Could you check a few things on this drawing? It's one solid part, dimensions in mm from its lowest x, y, z. A direction names the side the tool comes from. Give positions to 0.01 mm unless a question says otherwise; leave off trailing zeros. Loops run counter-clockwise (first coordinate to the right, second up) from the corner with the lowest first, then second, coordinate; pieces in that order, holes last. Notation, with made-up numbers: M 74.25,68 L 124.25,68 A20 ccw 124.25,82 Z; hole C 85.25,44.25 d4. An arc over 180 degrees is marked long. Answer as a JSON object with one key per item and string values.
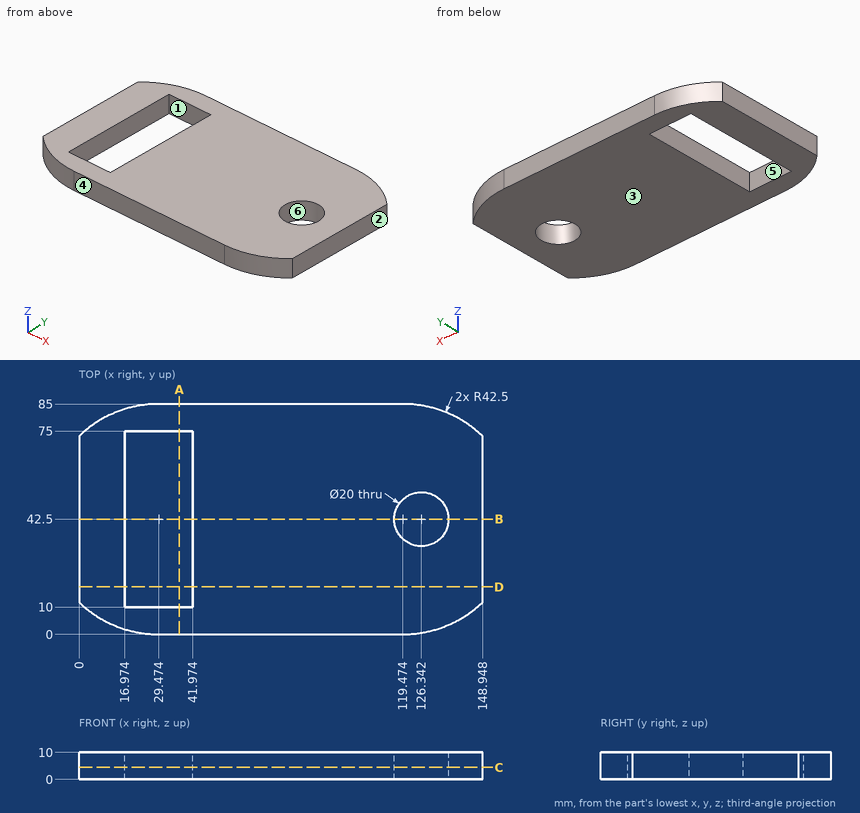
1) Will this pin go through, and if not, where does the flat tip stop? pin 1 Ø3 at (y, z) = (41.5, 7.5) entering from -X.
Answer list:
{"pin 1": "x = 0"}
2) Suppose I cut it at A-A, the plane x = 37. Write out the boundary of the cut face in (y, z).
Answer list:
{"outline": "M 0,0 L 10,0 L 10,10 L 0,10 Z; M 75,0 L 85,0 L 85,10 L 75,10 Z"}
3) Please list where these lines run through material, in increasing order: line 1 along X through (y, z) = (73, 1.75); line 2 along Y through (x, z) = (23, 3.25); line 3 along X through (y, z) = (48.5, 3) (1 decimal). Write a range as from..to.
Answer list:
{"line 1": "0..16.97, 41.97..148.95", "line 2": "0.5..10, 75..84.5", "line 3": "0..17, 42..118.3, 134.3..148.9"}
4) Suppose I cut it at D-D, the plane y = 17.5. Write out the boundary of the cut face in (x, z).
Answer list:
{"outline": "M 0,0 L 16.97,0 L 16.97,10 L 0,10 Z; M 41.97,0 L 148.95,0 L 148.95,10 L 41.97,10 Z"}
5) Suppose I cut it at C-C, the plane z = 4.5. Write out the boundary of the cut face in (x, y).
Answer list:
{"outline": "M 0,11.88 A42.5 ccw 29.47,0 L 119.47,0 A42.5 ccw 148.95,11.88 L 148.95,73.12 A42.5 ccw 119.47,85 L 29.47,85 A42.5 ccw 0,73.12 Z; hole M 16.97,10 L 41.97,10 L 41.97,75 L 16.97,75 Z; hole C 126.34,42.5 d20"}
6) For the marked faces 1 and 2, which set-ups out of +Z, -Z, +X, -X, +Y, -Y let a thin tool reach every point of the face, with its end or its side?
Answer list:
{"face 1": "+Z, -Z", "face 2": "+Z, -Z, +X, +Y, -Y"}
7) If we mould it in two halves opening along Y, with no side actions, what happens to the marked faces 3, 4, 5 and 6? For each: +Y half, -Y half, draft (parallel to the pull), parting line (faces both ways), or undercut.
Answer list:
{"face 3": "draft", "face 4": "-Y half", "face 5": "undercut", "face 6": "undercut"}
8) Suppose I cut it at B-B, the plane y = 42.5. Write out the boundary of the cut face in (x, z).
Answer list:
{"outline": "M 0,0 L 16.97,0 L 16.97,10 L 0,10 Z; M 41.97,0 L 116.34,0 L 116.34,10 L 41.97,10 Z; M 136.34,0 L 148.95,0 L 148.95,10 L 136.34,10 Z"}
